Part model, mm, in its own coordinate system. A direction names the side the tool comes from. Round coordinates to 2 decimals unless told otherwise and drop trailing zeros. Write each loop counter-clockwise with the first axis right and the second up, starting at its lowest first coordinate (ties: lowest second). Pieces come first, ordered by that corner, then holes.
```python
from build123d import *

# Parameters (mm, degrees)
SKETCH3_W               = 43.815
SKETCH3_H               = 87.63
SKETCH3_W_2             = 9.4615
SKETCH3_H_2             = 43.815
CUT_EXTRUDE1_DEPTH      = 15.875
HOLE1_D                 = 7.9248
HOLE1_DEPTH             = 23.58136
HOLE1_TIP               = 2.287692707
SKETCH8_R               = 3.2004
CUT_EXTRUDE2_DEPTH      = 7.096125
CUT_EXTRUDE2_DEPTH_BACK = 7.096125


with BuildPart() as part:
    # Sketch1 → Revolve1 (revolve)
    with BuildSketch(Plane.XY):
        Polygon((0, 0), (0, 8.90905), (0.762, 9.67105), (4.0386, 9.67105), (4.8006, 8.90905), (5.5626, 8.90905), (5.5626, 10.3759), (8.73633, 10.3759), (9.31418, 10.95375), (23.8506, 10.95375), (24.6126, 10.19175), (24.6126, 0), align=None)
    revolve(axis=Axis((24.6126, 0, 0), (-1, 0, 0)))

    # Sketch2 → Revolve2 (revolve)
    with BuildSketch(Plane.XY):
        with BuildLine():
            Line((24.6126, 0), (24.6126, 7.90575))
            Line((24.6126, 7.90575), (27.0002, 7.90575))
            Line((27.0002, 7.90575), (27.0002, 7.72795))
            ThreePointArc((27.0002, 7.72795), (27.260582072, 7.099332072), (27.8892, 6.83895))
            Line((27.8892, 6.83895), (29.1719, 6.83895))
            ThreePointArc((29.1719, 6.83895), (29.49290348, 6.898927826), (29.77059292, 7.0707683))
            Line((29.77059292, 7.0707683), (29.800517928, 7.09803))
            Line((29.800517928, 7.09803), (30.639987928, 7.9375))
            Line((30.639987928, 7.9375), (39.64813, 7.9375))
            Line((39.64813, 7.9375), (40.4876, 7.09803))
            Line((40.4876, 7.09803), (40.4876, 0))
            Line((40.4876, 0), (24.6126, 0))
        make_face()
    revolve(axis=Axis((40.4876, 0, 0), (-1, 0, 0)))

    # Sketch3 → Cut-Extrude1 (cut)
    with BuildSketch(Plane(origin=(40.4876, 0, 0), x_dir=(0, 0, -1), z_dir=(1, 0, 0))):
        Rectangle(SKETCH3_W, SKETCH3_H)
        Rectangle(SKETCH3_W_2, SKETCH3_H_2, mode=Mode.SUBTRACT)
    extrude(amount=-CUT_EXTRUDE1_DEPTH, mode=Mode.SUBTRACT)

    # Hole1
    with Locations(Plane.ZY):
        with Locations((0, 0)):
            Hole(HOLE1_D / 2, depth=HOLE1_DEPTH)
            with Locations((0, 0, -(HOLE1_DEPTH + HOLE1_TIP / 2))):  # 120° drill point
                Cone(0, HOLE1_D / 2, HOLE1_TIP, mode=Mode.SUBTRACT)

    # Sketch6 → Cut-Revolve1 (revolve, cut)
    with BuildSketch(Plane(origin=(0, 0, 0), x_dir=(1, 0, 0), z_dir=(0, 0.999847695, 0.017452406))):
        Polygon((17.4752, 0), (22.075197063, 0), (22.075197063, -3.28295), (22.314675925, -10.95375), (17.4752, -10.95375), align=None)
    revolve(axis=Axis((17.4752, -0.191169297, 10.952081691), (0, 0.017452406, -0.999847695)), mode=Mode.SUBTRACT)

    # Sketch7 → Revolve3 (revolve)
    with BuildSketch(Plane.XY):
        with BuildLine():
            Line((4.49554893, 10.291731804), (5.440112806, 9.347167928))
            ThreePointArc((5.440112806, 9.347167928), (5.477310245, 9.257365367), (5.440112806, 9.167562806))
            Line((5.440112806, 9.167562806), (5.1816, 8.90905))
            Line((5.1816, 8.90905), (4.8006, 8.90905))
            Line((4.8006, 8.90905), (4.8006, 8.65505))
            Line((4.8006, 8.65505), (5.5626, 8.65505))
            Line((5.5626, 8.65505), (5.5626, 9.51204893))
            Line((5.5626, 9.51204893), (4.69874893, 10.3759))
            Line((4.69874893, 10.3759), (4.49554893, 10.3759))
            Line((4.49554893, 10.3759), (4.49554893, 10.291731804))
        make_face()
    revolve(axis=Axis((5.5626, 0, 0), (-1, 0, 0)))

    # Sketch8 → Cut-Extrude2 (cut, two sides)
    with BuildSketch(Plane.XY) as cut_extrude2_sk:
        with Locations((33.3248, 0)):
            Circle(SKETCH8_R)
    extrude(amount=CUT_EXTRUDE2_DEPTH, mode=Mode.SUBTRACT)
    extrude(cut_extrude2_sk.sketch, amount=-CUT_EXTRUDE2_DEPTH_BACK, mode=Mode.SUBTRACT)


solid = part.part
```
Q1. Cut at A-A on x = 11.5. Write the cut outline in (y, z), plus the area to 3 significant figures.
Values follow:
outline: circle Ø21.91 at (0, 0); hole circle Ø7.92 at (0, 0)
area: 328 mm2
Q2. Drop flat-ended pins along their axis: pin 1 (2 mm diameter, centred on x = 31, y = 2.5, fed in from -Z); pin 2 (7.5 mm diameter, centred on x = 33.32, y = 0, fed in from +Z); pin 3 (1 mm diameter, centred on x = 24, z = 2.5, fed in from +Y). Give the stop position or say it passes through.
Values follow:
pin 1: stops at z = -4.73
pin 2: stops at z = 4.73
pin 3: stops at y = 10.77
Q3. Mould opens along Y. For faces 6 (the cylindrical face through (7.172, -10.366, -0.456)), 7 (the cylindrical face through (35.207, 7.937, 0.071)), 8 (the cylindrical face through (17.544, -4.634, 1.949)), 9 (the cylindrical face through (17.406, 4.563, 2.109)) say: +Y half, -Y half, draft (parallel to the pull), parting line (faces both ways), or undercut.
Values follow:
face 6: parting line
face 7: +Y half
face 8: undercut
face 9: undercut
Q4. Wall check: L1, parallel to Y at x = 14, z = -4; L2, parallel to Z at x = 30, y = -2.25; L3, parallel to X at y = -8.25, z = 0.75. Give the ranges that are in metal, low to high.
Values follow:
L1: y = -10.2 to 10.2
L2: z = -4.73 to 4.73
L3: x = 0 to 24.61
Q5. Which spindle directions (+Z, -Z, +X, -X, +Y, -Y) get a long thin tool onto all of the face, cutting with end or side? Do faces 1 (the flat face through (31, -3, 4.731)), 2 (the cylindrical face through (28.54, -6.84, -0.07)), 3 (the cylindrical face through (11.96, 1.19, -3.78)), 4 (the flat face through (31, -3, -4.731)), 5 (the conical face through (29.946, 7.243, 0.074)). Say none if no direction does.
Values follow:
face 1: +Z, +X, +Y, -Y
face 2: -Y
face 3: -X
face 4: -Z, +X, +Y, -Y
face 5: +Y
